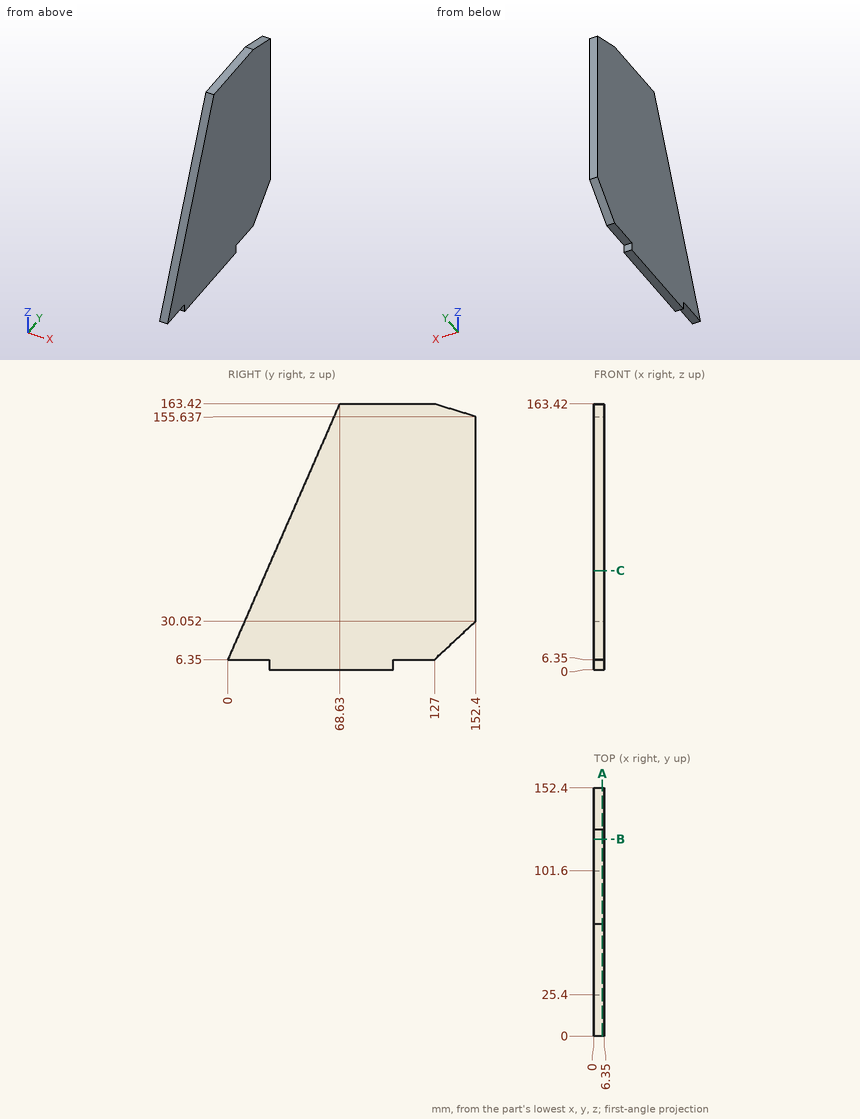
Part print with two shaded views. Sizes in mm from the minimum x, y, z corner. Round coordinates to 2 decimals unless told otherwise and drop trailing zeros. Order: outer loops, then holes, each group sorted by start corner. A loop starts at its lowest first (then second) coordinate and runs counter-clockwise, first axis right, second up. Notation, with made-up numbers: M -10.5,-28 L 8.5,-28 A31 cw 8.5,0 Z; hole C -21.5,-11.75 d7. An arc over 180 degrees is marked long. Use CSV: the item, a comma, the result in double quotes.
Item 1: Pin check, flat tips, straight feed: pin 1 (2 mm diameter, centred on x = 3, y = 133, fed in from -Z) (1 decimal); pin 2 (2 mm diameter, centred on x = 2, y = 125.5, fed in from -Z); pin 3 (2 mm diameter, centred on x = 1.5, y = 23, fed in from +Z) (1 decimal). Stop position of each tip, or through.
Worked answers:
pin 1,"z = 11"
pin 2,"z = 6.35"
pin 3,"z = 61.3"
Item 2: Probe probe 1 along Y at (x, z) = (1.25, 127.5) (1 decimal); probe 2 along Y at (x, z) = (3.5, 21); probe 3 along Z at (x, y) = (1.75, 37) (1 decimal). List the from-to ranges inside material, lowest first.
Worked answers:
probe 1,"52.9 to 152.4"
probe 2,"6.4 to 142.7"
probe 3,"0 to 91"
Item 3: Saw through at B-B (y = 121). List the corners of the cut face in (x, z).
Worked answers:
outline,"M 0,6.35 L 6.35,6.35 L 6.35,163.42 L 0,163.42 Z"
Item 4: Saw through at C-C (z = 61). List the corners of the cut face in (x, y).
Worked answers:
outline,"M 0,23.88 L 6.35,23.88 L 6.35,152.4 L 0,152.4 Z"
Item 5: Saw through at A-A (x = 5.25). List the corners of the cut face in (y, z), plus the area to 3 significant figures.
Worked answers:
outline,"M 0,6.35 L 25.4,6.35 L 25.4,0 L 101.6,0 L 101.6,6.35 L 127,6.35 L 152.4,30.05 L 152.4,155.64 L 127,163.42 L 68.63,163.42 Z"
area,"18,600 mm²"
